The listing builds one solid part. Answer for the finished solid, in the listing's coordinates (mm). A direction names the side the tool comes from. Give positions to 0.01 mm unless a question says otherwise; leave off trailing zeros. Order: outer loops, then holes, each group sorted by start corner. A loop starts at its lowest first (then second) coordinate and runs counter-clockwise, first axis right, second up. Notation, with made-up numbers: (44, 56.5) - (77, 56.5) arc R16 cw to (77, 63.5) - close; hole circle Ø11 at (-25.5, -4). An arc over 180 degrees is marked (long way). Answer as a JSON object with one key per item and string values. Group by question number.
Q1. Given pin 1 (2 mm diameter, centred on x = 20, z = 1101.5, fed in from +Y); pin 2 (3 mm diameter, centred on y = 7.5, z = 223, fed in from +X); pin 3 (12 mm diameter, centred on y = 12.5, z = 833, fed in from +X), each flat-ended and moving along its own axis, determine where each tip first touches the part or whether it passes through.
Q2. A cutting plane is placed at A-A, the plane z = 976. Give the vertices of the cut face in (x, y), and give its area (3 significant figures).
Q3. Consider line 1 (X direction, y = 23.5, z = 1188.5); line 2 (Y direction, x = 8, z = 364.5). Determine where each line is inside the solid, lowest interval first.
Q4. A cutting plane is placed at B-B, the plane x = 28. Give the vertices of the cut face in (y, z).
Q5. A cutting plane is placed at C-C, the plane y = 29.5. Give the vertices of the cut face in (x, z), and give its area (3 significant figures).
Q6. For faces 1 (the face through (0, 19, 614)), 2 (the face through (4.762, 23, 614)), determine the directions among +Z, -Z, +X, -X, +Y, -Y from which every point of the face is accessible in a straight line to the end or side of a thin tool.
Autodesk Inventor part; units mm, degrees
ref_plane "Start plane" through (0, 0, 0) normal (0, 0, 1) x (1, 0, 0)
ref_plane "End plane" through (0, 0, 1244.6) normal (0, 0, 1) x (1, 0, 0)
ref_plane "Work Plane4" through (19.05, 0, 1244.6) normal (0, 0.7071, 0.7071) x (1, 0, 0)
ref_plane "Start plane" through (0, 0, 0) normal (0, 0, 1) x (1, 0, 0)
ref_plane "End plane" through (0, 0, 1244.6) normal (0, 0, 1) x (1, 0, 0)
sketch "Sketch" plane through (0, 0, 0) normal (0, 0, 1) x (1, 0, 0)
  line L0 (38.1, 0) -> (0, 0)
  line L1 (0, 0) -> (0, 38.1)
  line L2 (0, 38.1) -> (2.4765, 38.1)
  line L3 (4.7625, 35.814) -> (4.7625, 9.5885)
  line L4 (9.5885, 4.7625) -> (35.814, 4.7625)
  line L5 (38.1, 2.4765) -> (38.1, 0)
  line L6 (0, -11.0414) -> (0, 31.5385) construction
  line L7 (-11.0414, 0) -> (31.5385, 0) construction
  arc A0 (4.7625, 9.5885) -> (9.5885, 4.7625) centre (9.5885, 9.5885) ccw
  arc A1 (4.7625, 35.814) -> (2.4765, 38.1) centre (2.4765, 35.814) ccw
  arc A2 (38.1, 2.4765) -> (35.814, 4.7625) centre (35.814, 2.4765) ccw
  line L8 (0, 48.4964) -> (0, -20.9644) construction
  line L9 (-20.9644, 0) -> (48.4964, 0) construction
  point P0 (4.7625, 38.1)
  point P1 (4.7625, 4.7625)
  point P2 (38.1, 4.7625)
  dimension "d0" = 38.1
  dimension "d1" = 38.1
  dimension "d2" = 4.7625
  dimension "d3" = 4.7625
  dimension "d10" = 0
  dimension "d11" = 0
  dimension "d14" = 4.826
  dimension "d15" = 2.286
extrude "Body" add sketch "Sketch" along normal up to surface (1244.6 mm away) from surface at 0
sketch "Sketch3" plane through (0, 0, 0) normal (0, 0, 1) x (1, 0, 0)
  line L0 (0, 0) -> (10, 0)
ref_plane "Work Plane3" through (0, 0, 0) normal (0, -1, 0) x (1, 0, 0)
sketch "Sketch4" plane through (0, 0, 0) normal (0, -1, 0) x (1, 0, 0)
  line L0 (-2, 0) -> (12, 0)
  line L1 (-2, 1244.6) -> (12, 1244.6)
  dimension "d17" = 1244.6
ref_plane "Work Plane4" through (19.05, 0, 1244.6) normal (0, 0.7071, 0.7071) x (1, 0, 0)
split "Split1" plane through (19.05, 0, 1244.6) removes the side toward (0, 0.7071, 0.7071)
ref_plane "Work Plane5" through (19.05, 0, 0) normal (0, 0.7071, -0.7071) x (1, 0, 0)
split "Split2" plane through (19.05, 0, 0) removes the side toward (0, 0.7071, -0.7071)
equation "\"d0\" = G_H"
equation "\"d1\" = G_H"
equation "\"d2\" = G_T"
equation "\"d3\" = G_T"
equation "\"d14\" = G_IR"
equation "\"d15\" = G_ER"
equation "\"d4\" = G_L"
equation "\"G_H\" = 38.1"
equation "\"G_T\" = 4.7625"
equation "\"G_ER\" = 2.286"
equation "\"G_IR\" = 4.826"
equation "\"G_L\" = d17"
equation "\"ex\" = 0"
equation "\"G_OFFSET_START\" = 0"
equation "\"G_OFFSET_END\" = 0"
equation "\"d13\" = G_OFFSET_END + B_L"
equation "\"B_L\" = 1244.6"
properties part number "AISC - L 1.5 x 1.5 x 3/16 - 49" material "Aluminum 6061"
Reply:
{
 "1": {"pin 1": "stops at y = 4.76", "pin 2": "stops at x = 6.36", "pin 3": "stops at x = 5.88"},
 "2": {"outline": "(0, 0) - (38.1, 0) - (38.1, 2.48) arc R2.29 ccw to (35.81, 4.76) - (9.59, 4.76) arc R4.83 cw to (4.76, 9.59) - (4.76, 35.81) arc R2.29 ccw to (2.48, 38.1) - (0, 38.1) - close", "area": "343 mm^2"},
 "3": {"line 1": "x = 0 to 4.76", "line 2": "y = 0 to 5.03"},
 "4": {"outline": "(0, 0) - (4.76, 4.76) - (4.76, 1239.84) - (0, 1244.6) - close"},
 "5": {"outline": "(0, 29.5) - (4.76, 29.5) - (4.76, 1215.1) - (0, 1215.1) - close", "area": "5,650 mm^2"},
 "6": {"face 1": "+Z, -Z, -X, +Y, -Y", "face 2": "+Z, -Z, +X, +Y"}
}
